Geometry check sheet. Reference: drawing and pictorial views, mm from the part's lowest x, y, z. A direction names the side the tool comes from. Round coordinates to 2 decimals unless told otherwise and drop trailing zeros. Loops run counter-clockwise (first coordinate to the right, second up) from the corner with the lowest first, then second, coordinate; pieces in that order, holes last. Notation, with made-up numbers: M 25,40 L 83,40 A19 cw 83,44 Z; hole C 39,85 d3. An arc over 180 degrees is marked long. One line per question, with ' | ' between items. Start each with the question number.
(1) Tool access check on the marked faces 1 and 2. Record the directions out of +Z, -Z, +X, -X, +Y, -Y that give a thin tool (end or side, any length) a straight path to the whole face; none if there is none.
(2) Draft check along X on the marked faces 3, 4, 5 and 6. Enter one of: +X half, -X half, draft (parallel to the pull), parting line (faces both ways), or undercut.
(3) Section check C-C (y = 53). Record the boundary of the cut face in (x, z).
(4) Go/stop test with flat-tipped pins: P1, Ø12, axis at x = 26.5, z = 6.5, coming from the +Y side; P2, Ø10, axis at x = 35.5, y = 48.5, coming from the +Z side; P3, Ø2.5, axis at y = 14.275, z = 20, coming from the +X side. Record where each tip stops, or that it passes through.
(5) Section check A-A (z = 20). Count the separate pieces of the cut face and the enclosed holes in it, and give its area (3 significant figures).
(6) Thickness scan on probe 1 along Y at (x, z) = (1.7, 20) (3 decimals); probe 2 along X at (y, z) = (56.5, 10); probe 3 along Z at (x, y) = (64, 17). Record the ranges inside material, lowest first. Write a range as [from, to].
(7) Section check D-D (x = 26). Record the boundary of the cut face in (y, z), and give its area (4 significant figures).
(8) Section check B-B (z = 13). Record the boundary of the cut face in (x, y), and give its area (3 significant figures).
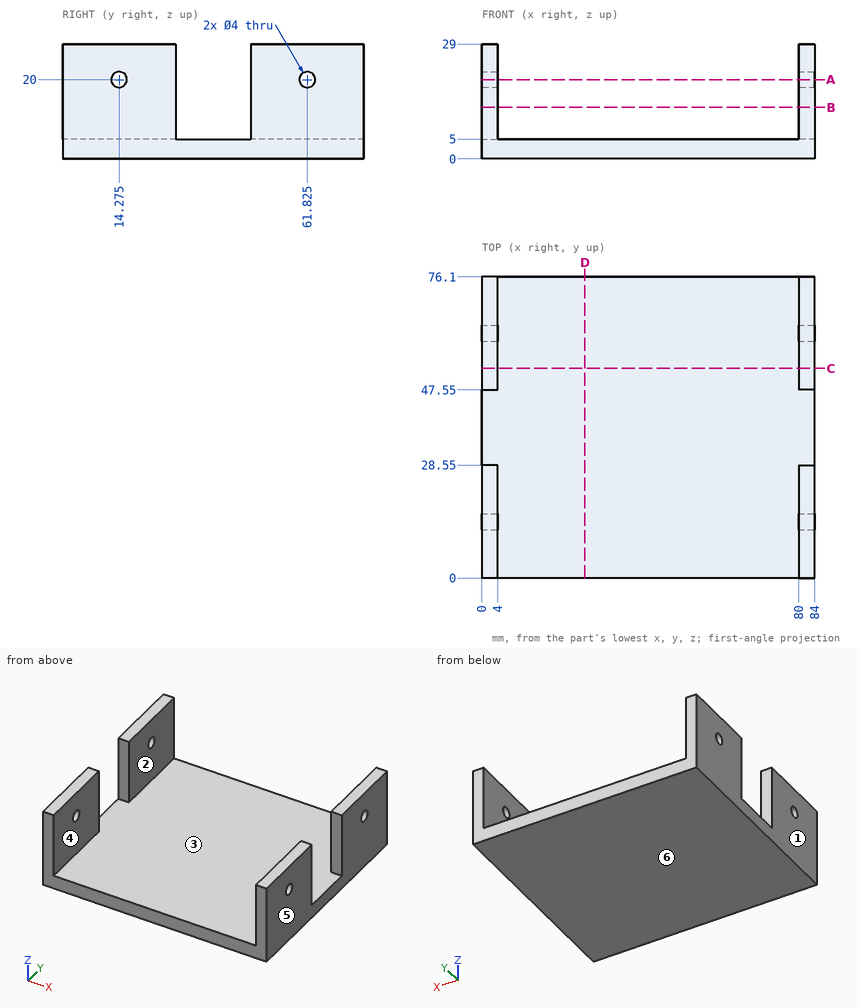
The answers:
1) face 1: +Z, -Z, -X, +Y, -Y | face 2: +Z, +Y, -Y
2) face 3: undercut | face 4: undercut | face 5: +X half | face 6: draft
3) outline: M 0,0 L 84,0 L 84,29 L 80,29 L 80,5 L 4,5 L 4,29 L 0,29 Z
4) P1: y = 76.1 | P2: z = 5 | P3: through
5) separate pieces: 8 | enclosed holes: 0 | area: 393 mm²
6) probe 1: [0, 12.275], [16.275, 28.55], [47.55, 59.825], [63.825, 76.1] | probe 2: [0, 4], [80, 84] | probe 3: [0, 5]
7) outline: M 0,0 L 76.1,0 L 76.1,5 L 0,5 Z | area: 380.5 mm²
8) outline: M 0,0 L 4,0 L 4,28.55 L 0,28.55 Z; M 0,47.55 L 4,47.55 L 4,76.1 L 0,76.1 Z; M 80,0 L 84,0 L 84,28.55 L 80,28.55 Z; M 80,47.55 L 84,47.55 L 84,76.1 L 80,76.1 Z | area: 457 mm²
